The model under review builds one solid part; all positions refer to its coordinate system, in mm. Give positions to 0.01 mm unless a question says otherwise; leave off trailing zeros. Order: outer loops, then holes, each group sorted by start corner. A loop starts at its lowest first (then second) coordinate and runs counter-clockwise, first axis right, second up. Notation, with made-up numbers: (-8, 77) - (39, 77) arc R26 ccw to (39, 111) - close; hole circle Ø1 at (56.5, 3). An arc over 180 degrees is marked (long way). Write item = value, one per line. Start each with the question number.
1. Wall thickness on probe 1 along X at (y, z) = (169, -90); probe 2 along Z at (x, y) = (224.5, 182); probe 3 along X at (y, z) = (20.5, -237.5): over which ranges is each line inside the solid? List them lowest first.
2. For P1, Ø10, axis at y = 176, z = -381.5, coming from the +X side, flat-tipped, find the tip position at first contact; note if it passes through.
3. We need section A-A, the plane x = 20.5. Give the boundary of the cut face in (y, z).
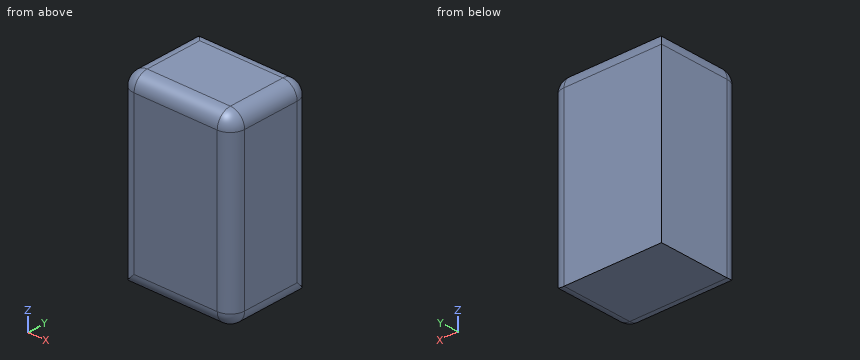
from build123d import *

# Parameters (mm, degrees)
F0_W     = 202.429667
F0_H     = 428.442776
F1_DEPTH = 262.275457
F3_R     = 33.614815


with BuildPart() as f1:
    # F0 (on Right) → F1 (new body)
    with BuildSketch(Plane.YZ):
        with Locations((101.214833, -214.221388)):
            Rectangle(F0_W, F0_H)
    extrude(amount=F1_DEPTH)

    # F3
    f3_edges = [f1.edges().sort_by_distance(p)[0] for p in [
        (262.275457, 101.214834, 0),
        (262.275457, 0, -214.221388),
        (262.275457, 101.214834, -428.442776),
        (262.275457, 202.429667, -214.221388),
        (131.137729, 0, 0),
        (131.137729, 0, -428.442776),
        (0, 0, -214.221388),
        (131.137729, 202.429667, 0),
        (0, 101.214834, 0),
    ]]
    fillet(f3_edges, radius=F3_R)


solid = f1.part
Model answer:
q1.probe_1 = 0 to 262.27
q1.probe_2 = -428.44 to -2.69
q1.probe_3 = 2.66 to 259.61
q2.P1 = 262.2
q3.outline = (2.66, -407.94) arc R33.61 ccw to (33.61, -428.44) - (202.43, -428.44) - (202.43, -33.61) arc R33.61 ccw to (181.93, -2.66) - (33.61, -2.66) arc R30.95 ccw to (2.66, -33.61) - close
